Could you check a few things on this model? Use its own coordinates, in mm. Face numbers are marked on the shaded views. Coordinates: 2 decimals unless noted, no trailing zeros. Order: outer loops, then holes, each group sorted by start corner. A loop starts at its lowest first (then second) coordinate and runs counter-clockwise, first axis right, second up. Notation, with made-up numbers: (49, 22) - (82, 22) arc R20 cw to (82, 27) - close; hole circle Ø5 at (31.5, 22.5). An arc over 180 degrees is marked (long way). Answer as a JSON object with one key per item and string values. Group by question number.
(1) Imagine slicing it at C-C, the plane x = 45. Write out the boundary of the cut face in (y, z), and give its area (3 significant figures).
(2) Please list where these lines run through material, in increasing order: probe 1 along Z at (x, y) = (20, -17.5); probe 2 along Y at (x, z) = (45, 1.6); probe 3 along Z at (x, y) = (38, 33.5).
(3) We'd pull the mould along Z, two halves only. Please class the marked faces 1, 2 and 3: pulls with the +Z half, pulls with the -Z half, needs draft (parallel to the pull), parting line crosses it, or undercut.
(4) Imagine slicing it at D-D, the plane x = -6.5. Write out the boundary of the cut face in (y, z), and give its area (3 significant figures).
(5) Imagine slicing it at B-B, the plane y = 1. Write out the boundary of the cut face in (x, z), and give its area (3 significant figures).
(6) Will these pins go through, and if not, where does the flat tip stop? P1, Ø2, axis at x = 63, z = 5, coming from the +Y side; P2, Ø4, axis at x = 10.5, y = 12, coming from the -Z side; P3, Ø1.8, axis at x = 44.5, y = 36.5, coming from the -Z side; P4, Ø1.1, axis at x = -49.5, z = 7.5, coming from the -Y side.
(7) Imagine slicing it at A-A, the plane z = 4.75. Write out the boundary of the cut face in (x, y).
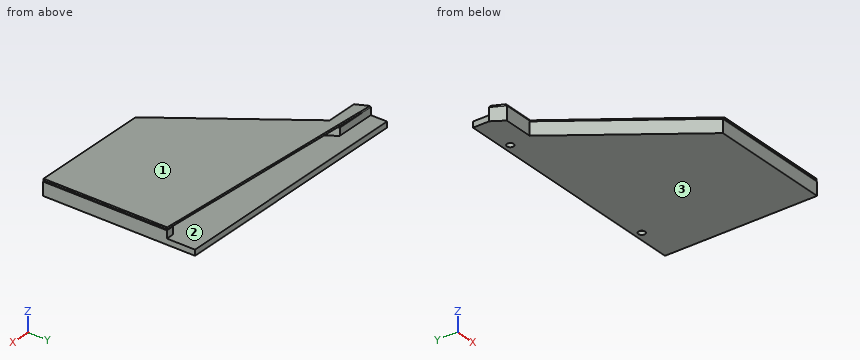
from build123d import *

# Parameters (mm, degrees)
PAD_DEPTH    = 3
SKETCH_R     = 1.75
POCKET_DEPTH = 2
PAD001_DEPTH = 4
PAD002_DEPTH = 1


with BuildPart() as part:
    # Sketch010 → Pad (new body)
    with BuildSketch(Plane.XY):
        Polygon((-46.128487, 25.244961), (1.34, -40), (65.75, -40), (65.75, 40), (-65.75, 40), (-65.75, 31.502308), (-61.754631, 25.244961), align=None)
    extrude(amount=PAD_DEPTH)

    # Sketch → Pocket (cut)
    with BuildSketch(Plane.XY):
        with Locations((-45, 36.301168)):
            Circle(SKETCH_R)
        with Locations((45, 36.301168)):
            Circle(SKETCH_R)
    extrude(amount=POCKET_DEPTH, mode=Mode.SUBTRACT)

    # Sketch011 (on Face5 of Pocket) → Pad001 (join)
    with BuildSketch(Plane.XY.offset(3)):
        Polygon((65.75, 25.244961), (65.75, -40), (1.34, -40), (-46.128487, 25.244961), (-61.754631, 25.244961), (-65.75, 31.502308), (-44.458256, 31.502308), (1.935629, -35.248356), (61.715927, -35.248356), (61.715927, 25.244961), align=None)
    extrude(amount=PAD001_DEPTH)

    # Sketch012 (on Face14 of Pad001) → Pad002 (join)
    with BuildSketch(Plane.XY.offset(7)):
        Polygon((-64.875565, 31.740883), (-61.877544, 25.56848), (-45.300247, 25.56848), (2.139057, -40.211658), (65.097519, -40.211658), (65.097519, 24.863066), align=None)
    extrude(amount=PAD002_DEPTH)


solid = part.part
Result set:
{
 "1": {"outline": "(-40.21, 7) - (-40, 7) - (-40, 0) - (34.55, 0) - (34.55, 2) - (38.05, 2) - (38.05, 0) - (40, 0) - (40, 3) - (-35.25, 3) - (-35.25, 7) - (25.93, 7) - (25.93, 8) - (-40.21, 8) - close", "area": "318 mm^2"},
 "2": {"probe 1": "z = 0 to 3, 7 to 8", "probe 2": "y = -40 to 34.55, 38.05 to 40", "probe 3": "z = 0 to 3"},
 "3": {"face 1": "pulls with the +Z half", "face 2": "undercut", "face 3": "pulls with the -Z half"},
 "4": {"outline": "(-29.22, 0) - (40, 0) - (40, 3) - (-23.11, 3) - (-23.11, 7) - (28.65, 7) - (28.65, 8) - (-28.23, 8) - (-28.23, 7) - (-29.22, 7) - close", "area": "289 mm^2"},
 "5": {"outline": "(-28.49, 0) - (65.75, 0) - (65.75, 7) - (65.1, 7) - (65.1, 8) - (-27.58, 8) - (-27.58, 7) - (-28.49, 7) - close; hole (-23.26, 3) - (61.72, 3) - (61.72, 7) - (-23.26, 7) - close", "area": "412 mm^2"},
 "6": {"P1": "stops at y = 25.24", "P2": "stops at z = 0", "P3": "stops at z = 2", "P4": "stops at y = 25.24"},
 "7": {"outline": "(-65.75, 31.5) - (-61.75, 25.24) - (-46.13, 25.24) - (1.34, -40) - (65.75, -40) - (65.75, 25.24) - (61.72, 25.24) - (61.72, -35.25) - (1.94, -35.25) - (-44.46, 31.5) - close"}
}
